Build history of the part. All positions in model axes, mm. Face numbers are marked on the shaded views. A direction names the side the tool comes from. Coordinates: 2 decimals unless noted, no trailing zeros. Loops run counter-clockwise (first coordinate to the right, second up) from the corner with the lowest first, then second, coordinate; pieces in that order, holes last. Notation, with made-up numbers: M 69.5,82 L 97.5,82 A16 ccw 97.5,113 Z; hole C 70.25,77 d1. An arc over 180 degrees is marked long. Write each question's results on one line, items separated by ' | '. Start each with the question number.
from build123d import *

# Parameters (mm, degrees)
F0_W     = 69.85
F0_H     = 38.1
F1_DEPTH = 25.4
F2_W     = 44.45
F2_H     = 25.4
F3_DEPTH = 25.401
F5_DEPTH = 25.401
F7_DEPTH = 12.701


with BuildPart() as f1:
    # F0 (on Front) → F1 (new body)
    with BuildSketch(Plane.XZ):
        with Locations((-3.4175124019, 11.064895078)):
            Rectangle(F0_W, F0_H)
    extrude(amount=F1_DEPTH)

    # F2 (on face) → F3 (cut, through all)
    with BuildSketch(Plane.XZ.offset(25.4)):
        with Locations((9.2824875981, 17.414895078)):
            Rectangle(F2_W, F2_H)
    extrude(amount=-F3_DEPTH, mode=Mode.SUBTRACT)

    # F4 (on face) → F5 (cut, through all)
    with BuildSketch(Plane.XZ.offset(25.4)):
        with BuildLine():
            Line((-19.2925124019, 30.114895078), (-19.2925124019, 28.7895729095))
            ThreePointArc((-19.2925124019, 28.7895729095), (-15.79175244, 26.6889172554), (-12.9425124019, 23.764895078))
            Line((-12.9425124019, 23.764895078), (-12.9425124019, 30.114895078))
            Line((-12.9425124019, 30.114895078), (-19.2925124019, 30.114895078))
        make_face()
        with BuildLine():
            Line((-38.3425124019, 30.114895078), (-38.3425124019, 23.764895078))
            ThreePointArc((-38.3425124019, 23.764895078), (-35.4932723639, 26.6889172554), (-31.9925124019, 28.7895729095))
            Line((-31.9925124019, 28.7895729095), (-31.9925124019, 30.114895078))
            Line((-31.9925124019, 30.114895078), (-38.3425124019, 30.114895078))
        make_face()
        with BuildLine():
            ThreePointArc((-19.2925124019, 17.414895078), (-21.1523843414, 21.9050231385), (-25.6425124019, 23.764895078))
            ThreePointArc((-25.6425124019, 23.764895078), (-30.1326404625, 21.9050231385), (-31.9925124019, 17.414895078))
            ThreePointArc((-31.9925124019, 17.414895078), (-30.132640455, 12.92476701), (-25.6425123807, 11.064895078))
            ThreePointArc((-25.6425123807, 11.064895078), (-21.1523843339, 12.924767025), (-19.2925124019, 17.414895078))
        make_face()
        with BuildLine():
            Line((-19.2925124019, 30.114895078), (-25.6425124019, 30.114895078))
            ThreePointArc((-25.6425124019, 30.114895078), (-22.3990968084, 29.7800327958), (-19.2925124019, 28.7895729095))
            Line((-19.2925124019, 28.7895729095), (-19.2925124019, 30.114895078))
        make_face()
        with BuildLine():
            Line((-31.9925124019, 30.114895078), (-31.9925124019, 28.7895729095))
            ThreePointArc((-31.9925124019, 28.7895729095), (-28.8859279955, 29.7800327958), (-25.6425124019, 30.114895078))
            Line((-25.6425124019, 30.114895078), (-31.9925124019, 30.114895078))
        make_face()
    extrude(amount=-F5_DEPTH, mode=Mode.SUBTRACT)

    # F6 (on face) → F7 (cut, through all)
    with BuildSketch(Plane.XY.offset(4.714895078)):
        with BuildLine():
            ThreePointArc((6.1074875981, -12.7), (4.2476156561, -8.209871937), (-0.242512409, -6.35))
            Line((-0.2425124019, -6.35), (-0.2425124019, -19.05))
            ThreePointArc((-0.2425123804, -19.05), (4.2476156662, -17.1901280529), (6.1074875981, -12.7))
        make_face()
        with BuildLine():
            Line((18.8074875981, -19.05), (18.8074875981, -6.35))
            ThreePointArc((18.8074875981, -6.35), (12.4574875981, -12.7), (18.8074875981, -19.05))
        make_face()
        with BuildLine():
            ThreePointArc((25.1574875981, -12.7), (23.2976156586, -8.2098719395), (18.8074875981, -6.35))
            Line((18.8074875981, -6.35), (18.8074875981, -19.05))
            ThreePointArc((18.8074875981, -19.05), (23.2976156586, -17.1901280605), (25.1574875981, -12.7))
        make_face()
        with BuildLine():
            Line((18.8074875981, -6.35), (-0.242512409, -6.35))
            ThreePointArc((-0.242512409, -6.35), (4.2476156561, -8.209871937), (6.1074875981, -12.7))
            ThreePointArc((6.1074875981, -12.7), (4.2476156662, -17.1901280529), (-0.2425123804, -19.05))
            Line((-0.2425123804, -19.05), (18.8074875981, -19.05))
            ThreePointArc((18.8074875981, -19.05), (12.4574875981, -12.7), (18.8074875981, -6.35))
        make_face()
        with BuildLine():
            Line((31.5074875981, 0), (18.8074875981, 0))
            ThreePointArc((18.8074875981, 0), (25.1574875981, -1.7014773719), (29.8060102261, -6.35))
            Line((29.8060102261, -6.35), (31.5074875981, -6.35))
            Line((31.5074875981, -6.35), (31.5074875981, 0))
        make_face()
        with BuildLine():
            ThreePointArc((29.8060102261, -19.05), (25.1574875981, -23.6985226281), (18.8074875981, -25.4))
            Line((18.8074875981, -25.4), (31.5074875981, -25.4))
            Line((31.5074875981, -25.4), (31.5074875981, -19.05))
            Line((31.5074875981, -19.05), (29.8060102261, -19.05))
        make_face()
        with BuildLine():
            Line((31.5074875981, -19.05), (31.5074875981, -12.7))
            ThreePointArc((31.5074875981, -12.7), (31.0747455919, -15.9870018728), (29.8060102261, -19.05))
            Line((29.8060102261, -19.05), (31.5074875981, -19.05))
        make_face()
        with BuildLine():
            Line((31.5074875981, -6.35), (29.8060102261, -6.35))
            ThreePointArc((29.8060102261, -6.35), (31.0747455919, -9.4129981272), (31.5074875981, -12.7))
            Line((31.5074875981, -12.7), (31.5074875981, -6.35))
        make_face()
        with BuildLine():
            Line((-0.2425124019, -19.05), (-0.2425124019, -6.35))
            ThreePointArc((-0.242512409, -6.35), (-6.5925124019, -12.7000000143), (-0.2425123804, -19.05))
        make_face()
    extrude(amount=-F7_DEPTH, mode=Mode.SUBTRACT)


solid = f1.part
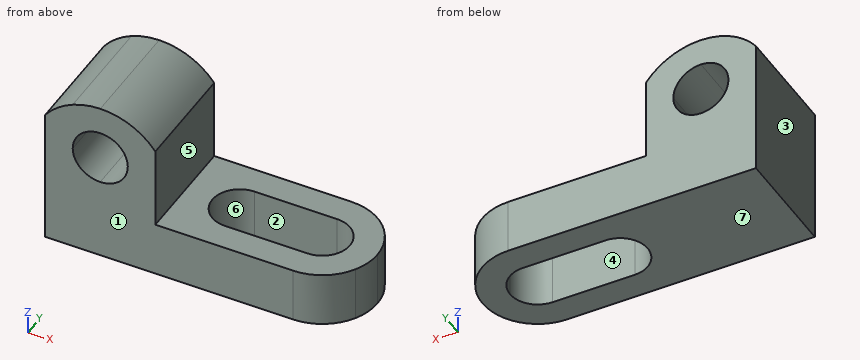
1. Wall check: line 1 along Z through (x, y) = (-26, -8.25); line 2 along X through (y, z) = (-22.75, 11); line 3 along Y through (x, z) = (12.5, -1.5). Give the ranges that are in metal, low to high.
2. Mould opens along Y. For the marked faces 1, 2, 3 and 4 say: +Y half, -Y half, draft (parallel to the pull), parting line (faces both ways), or undercut.
3. Pin check, flat tips, straight feed: pin 1 (6 mm diameter, centred on y = -20.5, z = -3, fed in from +X); pin 2 (1.5 mm diameter, centred on y = -15.5, z = 26, fed in from +X); pin 3 (1 mm diameter, centred on y = -14.5, z = 25, fed in from +X); pin 4 (4 mm diameter, centred on x = 19, y = -16, fed in from -Z). Stop position of each tip, or through.
4. Band-saw the part on D-D, the plane y = -23. List the corners of the cut face in (x, z) (3 decimals), plus the area to 3 significant figures.
5. Band-saw the part on A-A, the plane x = 16.5. List the corners of the cut face in (y, z).
6. Band-saw the part on B-B, the plane y = -9. List the corners of the cut face in (x, z) (3 decimals).
7. Which spindle directions (+Z, -Z, +X, -X, +Y, -Y) get a long thin tool onto all of the face, cutting with end or side? Do the marked faces 5, 6 and 7. Say none if no direction does.
8. Band-saw the part on C-C, the plane z = 0. List the corners of the cut face in (x, y).
Checked values:
1) line 1: -7.99 to 11.07, 23.75 to 30.11 | line 2: -38.34 to -12.94 | line 3: -25.4 to -19.05, -6.35 to 0
2) face 1: -Y half | face 2: undercut | face 3: draft | face 4: undercut
3) pin 1: x = 30.57 | pin 2: x = -14.21 | pin 3: x = -13.53 | pin 4: through
4) outline: M -38.343,-7.985 L 26.237,-7.985 L 26.237,4.715 L -12.943,4.715 L -12.943,23.765 A15.875 ccw -38.343,23.765 Z; hole C -25.643,17.415 d12.7 | area: 1,290 mm²
5) outline: M -25.4,-7.99 L -19.05,-7.99 L -19.05,4.71 L -25.4,4.71 Z; M -6.35,-7.99 L 0,-7.99 L 0,4.71 L -6.35,4.71 Z
6) outline: M -38.343,-7.985 L -5.403,-7.985 L -5.403,4.715 L -12.943,4.715 L -12.943,23.765 A15.875 ccw -38.343,23.765 Z; M 23.968,-7.985 L 30.957,-7.985 L 30.957,4.715 L 23.968,4.715 Z; hole C -25.643,17.415 d12.7
7) face 5: +Z, +X, +Y, -Y | face 6: +Z, -Z | face 7: -Z, +X, -X, +Y, -Y
8) outline: M -38.34,-25.4 L 18.81,-25.4 A12.7 ccw 18.81,0 L -38.34,0 Z; hole M -0.24,-19.05 L 18.81,-19.05 A6.35 ccw 18.81,-6.35 L -0.24,-6.35 A6.35 ccw Z
